```python
from build123d import *

# Parameters (mm, degrees)
SKETCH1_W             = 25.4
SKETCH1_H             = 25.4
BOSS_EXTRUDE1_DEPTH   = 56.75
SKETCH2_W             = 23.8125
SKETCH2_H             = 23.8125
CUT_EXTRUDE1_DEPTH    = 115.912270885
FILLET1_R             = 0.508
M3_CLEARANCE_HOLE1_D  = 3.4
M3_CLEARANCE_HOLE2_D  = 3.4
M3_CLEARANCE_HOLE3_D  = 3.4
M3_CLEARANCE_HOLE4_D  = 3.4
FILLET2_R             = 1.5
CUT_EXTRUDE2_REACH    = 65.459
SKETCH11_W            = 16.9
SKETCH11_H            = 6.499999954
SKETCH11_H_2          = 7
CUT_EXTRUDE3_REACH    = 65.459
SKETCH12_W            = 16.9
SKETCH12_H            = 6.5
SKETCH12_H_2          = 7
FILLET3_R             = 3.81
CUT_EXTRUDE4_REACH    = 65.459
SKETCH13_W            = 15.4
SKETCH13_H            = 87.3
CUT_EXTRUDE5_REACH    = 65.459
SKETCH14_W            = 15.4
SKETCH14_H            = 87.3
CHAMFER2_SIZE         = 6.35
FILLET5_R             = 3.81
SKETCH15_W            = 12.31
SKETCH15_H            = 12.31
CUT_EXTRUDE6_DEPTH    = 6.5
SKETCH17_W            = 12.31
SKETCH17_H            = 12.31
CUT_EXTRUDE8_DEPTH    = 7
BOSS_EXTRUDE2_START   = -1.5875
BOSS_EXTRUDE2_DEPTH   = 1.5875
BOSS_EXTRUDE3_START   = -1.5875
BOSS_EXTRUDE3_DEPTH   = 1.5875
CUT_EXTRUDE12_REACH   = 59.038
SKETCH23_W            = 6.5
SKETCH23_H            = 7
FILLET9_R             = 1.5875
FILLET9_OF_MIRROR3_R  = 1.5875
BOSS_EXTRUDE4_DEPTH   = 1.5875
SKETCH25_W            = 9
SKETCH25_H            = 9
CUT_EXTRUDE13_DEPTH   = 2
FILLET10_R            = 0.5
FILLET10_OF_MIRROR4_R = 0.5


with BuildPart() as part:
    # Sketch1 → Boss-Extrude1 (new, symmetric)
    with BuildSketch(Plane(origin=(0, 0, 0), x_dir=(1, 0, 0), z_dir=(0, 1, 0))):
        Rectangle(SKETCH1_W, SKETCH1_H)
    extrude(amount=BOSS_EXTRUDE1_DEPTH, both=True)

    # Sketch2 → Cut-Extrude1 (cut, through all)
    with BuildSketch(Plane(origin=(0, 56.75, 0), x_dir=(1, 0, 0), z_dir=(0, 1, 0))):
        with Locations((0.79375, 0.79375)):
            Rectangle(SKETCH2_W, SKETCH2_H)
    extrude(amount=-CUT_EXTRUDE1_DEPTH, mode=Mode.SUBTRACT)

    # Fillet1
    fillet1_edges = [part.edges().sort_by_distance(p)[0] for p in [
        (-11.1125, 0, 11.1125),
    ]]
    fillet(fillet1_edges, radius=FILLET1_R)

    # M3 Clearance Hole1 (through all)
    with Locations(Plane.XY.offset(12.7)):
        with Locations((6.35, 47.075)):
            Hole(M3_CLEARANCE_HOLE1_D / 2)

    # M3 Clearance Hole2 (through all)
    with Locations(Plane.ZY.offset(12.7)):
        with Locations((-6.35, 47.075)):
            Hole(M3_CLEARANCE_HOLE2_D / 2)

    # M3 Clearance Hole3 (through all)
    with Locations(Plane.XY.offset(12.7)):
        with Locations((6.35, -46.575)):
            Hole(M3_CLEARANCE_HOLE3_D / 2)

    # M3 Clearance Hole4 (through all)
    with Locations(Plane.ZY.offset(12.7)):
        with Locations((-6.35, -46.575)):
            Hole(M3_CLEARANCE_HOLE4_D / 2)

    # Fillet2
    fillet2_edges = [part.edges().sort_by_distance(p)[0] for p in [
        (-12.7, 0, 12.7),
    ]]
    fillet(fillet2_edges, radius=FILLET2_R)

    # Sketch11 → Cut-Extrude2 (cut, up to next)
    with BuildSketch(Plane.ZY.offset(12.7), mode=Mode.PRIVATE) as cut_extrude2_sk1:
        with Locations((-4.25, 53.500000023)):
            Rectangle(SKETCH11_W, SKETCH11_H)
    cut_extrude2_tool1 = extrude(cut_extrude2_sk1.sketch, amount=-CUT_EXTRUDE2_REACH, mode=Mode.PRIVATE) & part.part
    # Sketch11 → Cut-Extrude2 (cut, up to next)
    with BuildSketch(Plane.ZY.offset(12.7), mode=Mode.PRIVATE) as cut_extrude2_sk2:
        with Locations((-4.25, -53.25)):
            Rectangle(SKETCH11_W, SKETCH11_H_2)
    cut_extrude2_tool2 = extrude(cut_extrude2_sk2.sketch, amount=-CUT_EXTRUDE2_REACH, mode=Mode.PRIVATE) & part.part
    add(cut_extrude2_tool1.solids().sort_by_distance((-12.7, 53.5, -4.25))[0], mode=Mode.SUBTRACT)
    add(cut_extrude2_tool2.solids().sort_by_distance((-12.7, -53.25, -4.25))[0], mode=Mode.SUBTRACT)

    # Sketch12 → Cut-Extrude3 (cut, up to next)
    with BuildSketch(Plane.XY.offset(12.7), mode=Mode.PRIVATE) as cut_extrude3_sk1:
        with Locations((4.25, 53.5)):
            Rectangle(SKETCH12_W, SKETCH12_H)
    cut_extrude3_tool1 = extrude(cut_extrude3_sk1.sketch, amount=-CUT_EXTRUDE3_REACH, mode=Mode.PRIVATE) & part.part
    # Sketch12 → Cut-Extrude3 (cut, up to next)
    with BuildSketch(Plane.XY.offset(12.7), mode=Mode.PRIVATE) as cut_extrude3_sk2:
        with Locations((4.25, -53.25)):
            Rectangle(SKETCH12_W, SKETCH12_H_2)
    cut_extrude3_tool2 = extrude(cut_extrude3_sk2.sketch, amount=-CUT_EXTRUDE3_REACH, mode=Mode.PRIVATE) & part.part
    add(cut_extrude3_tool1.solids().sort_by_distance((4.25, 53.5, 12.7))[0], mode=Mode.SUBTRACT)
    add(cut_extrude3_tool2.solids().sort_by_distance((4.25, -53.25, 12.7))[0], mode=Mode.SUBTRACT)

    # Fillet3
    fillet3_edges = [part.edges().sort_by_distance(p)[0] for p in [
        (-4.2, 50.25, 11.90625),
        (-4.2, -49.75, 11.90625),
        (-11.90625, 50.250000046, 4.2),
        (-11.90625, -49.75, 4.2),
    ]]
    fillet(fillet3_edges, radius=FILLET3_R)

    # Sketch13 → Cut-Extrude4 (cut, up to next)
    with BuildSketch(Plane.ZY.offset(12.7), mode=Mode.PRIVATE) as cut_extrude4_sk1:
        with Locations((-5, 0.25)):
            Rectangle(SKETCH13_W, SKETCH13_H)
    cut_extrude4_tool1 = extrude(cut_extrude4_sk1.sketch, amount=-CUT_EXTRUDE4_REACH, mode=Mode.PRIVATE) & part.part
    add(cut_extrude4_tool1.solids().sort_by_distance((-12.7, 0.25, -5))[0], mode=Mode.SUBTRACT)

    # Sketch14 → Cut-Extrude5 (cut, up to next)
    with BuildSketch(Plane.XY.offset(12.7), mode=Mode.PRIVATE) as cut_extrude5_sk1:
        with Locations((5, 0.25)):
            Rectangle(SKETCH14_W, SKETCH14_H)
    cut_extrude5_tool1 = extrude(cut_extrude5_sk1.sketch, amount=-CUT_EXTRUDE5_REACH, mode=Mode.PRIVATE) & part.part
    add(cut_extrude5_tool1.solids().sort_by_distance((5, 0.25, 12.7))[0], mode=Mode.SUBTRACT)

    # Chamfer2
    chamfer2_edges = [part.edges().sort_by_distance(p)[0] for p in [
        (-11.90625, 43.9, 2.7),
        (-11.90625, -43.4, 2.7),
        (-2.7, -43.4, 11.90625),
        (-2.7, 43.9, 11.90625),
    ]]
    chamfer(chamfer2_edges, length=CHAMFER2_SIZE)

    # Fillet5
    fillet5_edges = [part.edges().sort_by_distance(p)[0] for p in [
        (-11.90625, 43.9, -3.65),
        (-11.90625, -37.05, 2.7),
        (-11.90625, 37.55, 2.7),
        (-2.7, -37.05, 11.90625),
        (-2.7, 37.55, 11.90625),
        (3.65, 43.9, 11.90625),
        (3.65, -43.4, 11.90625),
        (-11.90625, -43.4, -3.65),
    ]]
    fillet(fillet5_edges, radius=FILLET5_R)

    # Sketch15 → Cut-Extrude6 (cut)
    with BuildSketch(Plane(origin=(0, 56.75, 0), x_dir=(1, 0, 0), z_dir=(0, 1, 0))):
        with Locations((-6.545, -6.545)):
            Rectangle(SKETCH15_W, SKETCH15_H)
    extrude(amount=-CUT_EXTRUDE6_DEPTH, mode=Mode.SUBTRACT)

    # Sketch17 → Cut-Extrude8 (cut)
    with BuildSketch(Plane.XZ.offset(56.75)):
        with Locations((-6.545, 6.545)):
            Rectangle(SKETCH17_W, SKETCH17_H)
    extrude(amount=-CUT_EXTRUDE8_DEPTH, mode=Mode.SUBTRACT)

    # Sketch20 → Boss-Extrude2 (add)
    with BuildSketch(Plane.ZY.offset(12.7).offset(BOSS_EXTRUDE2_START)):
        with BuildLine():
            Line((-12.7, 43.9), (-12.7, -43.4))
            Line((-12.7, -43.4), (-5.228153673, -43.4))
            ThreePointArc((-5.228153673, -43.4), (-3.770129795, -43.109981019), (-2.534076836, -42.284076836))
            Line((-2.534076836, -42.284076836), (1.584076836, -38.165923164))
            ThreePointArc((1.584076836, -38.165923164), (2.409981019, -36.929870205), (2.7, -35.471846327))
            Line((2.7, -35.471846327), (2.7, 35.971846327))
            ThreePointArc((2.7, 35.971846327), (2.409981019, 37.429870205), (1.584076836, 38.665923164))
            Line((1.584076836, 38.665923164), (-2.534076836, 42.784076836))
            ThreePointArc((-2.534076836, 42.784076836), (-3.770129795, 43.609981019), (-5.228153673, 43.9))
            Line((-5.228153673, 43.9), (-12.7, 43.9))
        make_face()
    extrude(amount=BOSS_EXTRUDE2_DEPTH)

    # Sketch21 → Boss-Extrude3 (add)
    with BuildSketch(Plane.XY.offset(12.7).offset(BOSS_EXTRUDE3_START)):
        with BuildLine():
            Line((12.7, 43.9), (12.7, -43.4))
            Line((12.7, -43.4), (5.228153673, -43.4))
            ThreePointArc((5.228153673, -43.4), (3.770129795, -43.109981019), (2.534076836, -42.284076836))
            Line((2.534076836, -42.284076836), (-1.584076836, -38.165923164))
            ThreePointArc((-1.584076836, -38.165923164), (-2.409981019, -36.929870205), (-2.7, -35.471846327))
            Line((-2.7, -35.471846327), (-2.7, 35.971846327))
            ThreePointArc((-2.7, 35.971846327), (-2.409981019, 37.429870205), (-1.584076836, 38.665923164))
            Line((-1.584076836, 38.665923164), (2.534076836, 42.784076836))
            ThreePointArc((2.534076836, 42.784076836), (3.770129795, 43.609981019), (5.228153673, 43.9))
            Line((5.228153673, 43.9), (12.7, 43.9))
        make_face()
    extrude(amount=BOSS_EXTRUDE3_DEPTH)

    # Sketch23 → Cut-Extrude12 (cut, up to next)
    with BuildSketch(Plane(origin=(-11.1125, 0, 0), x_dir=(0, 0, -1), z_dir=(1, 0, 0)), mode=Mode.PRIVATE) as cut_extrude12_sk1:
        with Locations((-5.8625, 37.75)):
            Rectangle(SKETCH23_W, SKETCH23_H)
    cut_extrude12_tool1 = extrude(cut_extrude12_sk1.sketch, amount=-CUT_EXTRUDE12_REACH, mode=Mode.PRIVATE) & part.part
    cut_extrude12 = cut_extrude12_tool1.solids().sort_by_distance((-11.1125, 37.75, 5.8625))[0]
    add(cut_extrude12, mode=Mode.SUBTRACT)

    # Fillet9
    fillet9_edges = [part.edges().sort_by_distance(p)[0] for p in [
        (-11.90625, 41.25, 9.1125),
        (-11.90625, 41.25, 2.6125),
        (-11.90625, 34.25, 2.6125),
        (-11.90625, 34.25, 9.1125),
    ]]
    fillet(fillet9_edges, radius=FILLET9_R)

    # Mirror3: Cut-Extrude12 across plane
    add(cut_extrude12.mirror(Plane.ZX.offset(0.250000023)), mode=Mode.SUBTRACT)

    # Fillet9 of Mirror3
    fillet9_of_mirror3_edges = [part.edges().sort_by_distance(p)[0] for p in [
        (-11.90625, -40.749999954, 9.1125),
        (-11.90625, -40.749999954, 2.6125),
        (-11.90625, -33.749999954, 2.6125),
        (-11.90625, -33.749999954, 9.1125),
    ]]
    fillet(fillet9_of_mirror3_edges, radius=FILLET9_OF_MIRROR3_R)

    # Sketch24 → Boss-Extrude4 (add)
    with BuildSketch(Plane.ZY.offset(12.7)):
        with BuildLine():
            Line((4.2, 34.25), (7.525, 34.25))
            ThreePointArc((7.525, 34.25), (8.647532015, 34.714967985), (9.1125, 35.8375))
            Line((9.1125, 35.8375), (9.1125, 39.6625))
            ThreePointArc((9.1125, 39.6625), (8.647532015, 40.785032015), (7.525, 41.25))
            Line((7.525, 41.25), (4.2, 41.25))
            ThreePointArc((4.2, 41.25), (3.077467985, 40.785032015), (2.6125, 39.6625))
            Line((2.6125, 39.6625), (2.6125, 35.8375))
            ThreePointArc((2.6125, 35.8375), (3.077467985, 34.714967985), (4.2, 34.25))
        make_face()
    extrude(amount=-BOSS_EXTRUDE4_DEPTH)

    # Sketch25 → Cut-Extrude13 (cut)
    with BuildSketch(Plane.XZ.offset(49.75)):
        with Locations((-8.2, 8.2)):
            Rectangle(SKETCH25_W, SKETCH25_H)
    cut_extrude13 = extrude(amount=-CUT_EXTRUDE13_DEPTH, mode=Mode.SUBTRACT)

    # Fillet10
    fillet10_edges = [part.edges().sort_by_distance(p)[0] for p in [
        (-3.7, -47.75, 11.90625),
        (-11.90625, -47.75, 3.7),
    ]]
    fillet(fillet10_edges, radius=FILLET10_R)

    # Mirror4: Cut-Extrude13 across plane
    add(cut_extrude13.mirror(Plane.ZX.offset(0.250000023)), mode=Mode.SUBTRACT)

    # Fillet10 of Mirror4
    fillet10_of_mirror4_edges = [part.edges().sort_by_distance(p)[0] for p in [
        (-3.7, 48.250000046, 11.90625),
        (-11.90625, 48.250000046, 3.7),
    ]]
    fillet(fillet10_of_mirror4_edges, radius=FILLET10_OF_MIRROR4_R)


solid = part.part
```
For this review, take the finished solid that the model builds, in its own axes (mm). A direction names the side the tool comes from. Coordinates: 2 decimals unless noted, no trailing zeros. Loops run counter-clockwise (first coordinate to the right, second up) from the corner with the lowest first, then second, coordinate; pieces in that order, holes last. Notation, with made-up numbers: (15.25, 83.25) - (21.25, 83.25) arc R15 cw to (21.25, 106.25) - close; hole circle Ø3 at (-29, -12). An arc over 180 degrees is marked (long way). Use one line per item in the form item = value. Start each with the question number.
1) For pin 1 (0.5 mm diameter, centred on x = -12, z = 6, fed in from +Y); pin 2 (1.2 mm diameter, centred on y = -49, z = 11.5, fed in from -X); pin 3 (5 mm diameter, centred on y = 3, z = 9.5, fed in from +X); pin 4 (8 mm diameter, centred on x = 5, y = 39, fed in from -Z), all flat-tipped, find the tip position at first contact; note any pin that passes through.
2) Draft analysis for pull direction Y (two halves, no side actions). For faces 1 (the face through (-9.5, 48.25, 11.3)), 2 (the face through (1, 1, 12.7)), 3 (the face through (-11.895, -45.426, -5.097)), state which applies: released by +Y, released by -Y, zero draft, split by the parting line, or undercut.
3) For faces 4 (the face through (-11.895, 45.415, -5.981)), 5 (the face through (-9.5, -47.75, 11.3)), 6 (the face through (-11.112, 1, -1)), list the 3-axis set-ups (+Z, -Z, +X, -X, +Y, -Y) from which the entire face can be reached by the end or side of a thin tool; tool diameter is ignored.
4) Take a section at C-C (z = 6.25). State the section outline as (x, y) points.
5) Take a section at D-D (x = 10.75). State the section outline as (y, z) points.
6) To check wall thickness, follow probe 1 along Y at (x, z) = (6.35, 12.05) (3 decimals); probe 2 along X at (y, z) = (-26, 3.5); probe 3 along Z at (x, y) = (-8, 39). State the ranges of each line that lie inside material, in increasing order. Write a range as from..to.
7) Take a section at A-A (z = -6.35). State how many separate pieces and enclosed holes the cut face has, plus the area to 3 significant figures.
From the geometry:
q1.pin_1 = 48.25
q1.pin_2 = -3.7
q1.pin_3 = 12.7
q1.pin_4 = 11.11
q2.face_1 = released by +Y
q2.face_2 = zero draft
q2.face_3 = undercut
q3.face_4 = +X, -X
q3.face_5 = +Z, -X, -Y
q3.face_6 = -Z, +X, +Y, -Y
q4.outline = (-12.7, -47.75) - (-11.11, -47.75) - (-11.11, -40.75) - (-12.7, -40.75) - close; (-12.7, -33.75) - (-11.11, -33.75) - (-11.11, 48.25) - (-12.7, 48.25) - close
q5.outline = (-49.75, 11.11) - (50.25, 11.11) - (50.25, 12.7) - (-49.75, 12.7) - close
q6.probe_1 = -49.75..-48.275, -44.875..45.375, 48.775..50.25
q6.probe_2 = -12.7..-11.11
q6.probe_3 = 11.11..12.7
q7.separate_pieces = 3
q7.enclosed_holes = 0
q7.area = 148 mm2
